from build123d import *

# Parameters (mm, degrees)
SKIZZE1_W                               = 80
SKIZZE1_H                               = 46
SKIZZE1_R                               = 5
SKIZZE1_R_2                             = 1
AUFSATZ_LINEAR_AUSTRAGEN1_DEPTH         = 3
AUFSATZ_LINEAR_AUSTRAGEN1_DEPTH_BACK    = 3
F_3_0_3_DURCHMESSER_BOHRUNG1_AT_2_COUNT = 2
F_3_0_3_DURCHMESSER_BOHRUNG1_AT_2_PITCH = 40
SKIZZE4_W                               = 32
SKIZZE4_H                               = 46
SCHNITT_LINEAR_AUSTRAGEN1_DEPTH         = 4
SCHNITT_LINEAR_AUSTRAGEN3_DEPTH         = 4.5
SKIZZE9_W                               = 35.5
SKIZZE9_H                               = 44
SCHNITT_LINEAR_AUSTRAGEN5_DEPTH         = 2
AUFSATZ_LINEAR_AUSTRAGEN2_DEPTH         = 34
FASE1_SIZE                              = 0.7


with BuildPart() as part:
    # Skizze1 → Aufsatz-Linear austragen1 (new body, two sides)
    with BuildSketch(Plane.XY) as aufsatz_linear_austragen1_sk:
        Rectangle(SKIZZE1_W, SKIZZE1_H)
        with Locations((0, -12)):
            Circle(SKIZZE1_R, mode=Mode.SUBTRACT)
        with Locations((0, -2)):
            Circle(SKIZZE1_R_2, mode=Mode.SUBTRACT)
    extrude(amount=AUFSATZ_LINEAR_AUSTRAGEN1_DEPTH)
    extrude(aufsatz_linear_austragen1_sk.sketch, amount=-AUFSATZ_LINEAR_AUSTRAGEN1_DEPTH_BACK)

    # Skizze2 → Ø3.0 (3) Durchmesser Bohrung1 (revolve, cut)
    with BuildSketch(Plane(origin=(40, -20, 0), x_dir=(0, 0, -1), z_dir=(0, 1, 0))):
        Polygon((0, 0), (0, 12.901290929), (1.5, 12), (1.5, 0), align=None)
    f_3_0_3_durchmesser_bohrung1 = revolve(axis=Axis((46.35, -20, 0), (-1, 0, 0)), mode=Mode.SUBTRACT)

    # Ø3.0 (3) Durchmesser Bohrung1 at 2: Ø3.0 (3) Durchmesser Bohrung1 ×2
    with Locations(*[(0, i * F_3_0_3_DURCHMESSER_BOHRUNG1_AT_2_PITCH, 0) for i in range(1, F_3_0_3_DURCHMESSER_BOHRUNG1_AT_2_COUNT)]):
        add(f_3_0_3_durchmesser_bohrung1, mode=Mode.SUBTRACT)

    # Spiegeln1: Ø3.0 (3) Durchmesser Bohrung1 across plane
    add(f_3_0_3_durchmesser_bohrung1.mirror(Plane(origin=(0, 0, 0), x_dir=(0, 0, 1), z_dir=(1, 0, 0))), mode=Mode.SUBTRACT)

    # Spiegeln1 copy 1 sketch → Spiegeln1 copy 1 (revolve, cut)
    with BuildSketch(Plane(origin=(-40, 20, 0), x_dir=(0, 0, -1), z_dir=(0, 1, 0))):
        Polygon((0, 0), (0, -12.901290929), (1.5, -12), (1.5, 0), align=None)
    revolve(axis=Axis((-46.35, 20, 0), (-1, 0, 0)), mode=Mode.SUBTRACT)

    # Skizze4 → Schnitt-Linear austragen1 (cut)
    with BuildSketch(Plane.XY.offset(-3)):
        Rectangle(SKIZZE4_W, SKIZZE4_H)
    extrude(amount=SCHNITT_LINEAR_AUSTRAGEN1_DEPTH, mode=Mode.SUBTRACT)

    # Skizze6 → Schnitt-Linear austragen3 (cut)
    with BuildSketch(Plane(origin=(0, 0, -3), x_dir=(-1, 0, 0), z_dir=(0, 0, -1))):
        with BuildLine():
            Line((37, 15), (37, -15))
            ThreePointArc((37, -15), (36.414213562, -16.414213562), (35, -17))
            Line((35, -17), (22, -17))
            ThreePointArc((22, -17), (20.585786438, -16.414213562), (20, -15))
            Line((20, -15), (20, 15))
            ThreePointArc((20, 15), (20.585786438, 16.414213562), (22, 17))
            Line((22, 17), (35, 17))
            ThreePointArc((35, 17), (36.414213562, 16.414213562), (37, 15))
        make_face()
        with BuildLine():
            Line((-35, 17), (-22, 17))
            ThreePointArc((-22, 17), (-20.585786438, 16.414213562), (-20, 15))
            Line((-20, 15), (-20, -15))
            ThreePointArc((-20, -15), (-20.585786438, -16.414213562), (-22, -17))
            Line((-22, -17), (-35, -17))
            ThreePointArc((-35, -17), (-36.414213562, -16.414213562), (-37, -15))
            Line((-37, -15), (-37, 15))
            ThreePointArc((-37, 15), (-36.414213562, 16.414213562), (-35, 17))
        make_face()
    extrude(amount=-SCHNITT_LINEAR_AUSTRAGEN3_DEPTH, mode=Mode.SUBTRACT)

    # Skizze9 → Schnitt-Linear austragen5 (cut)
    with BuildSketch(Plane(origin=(0, 0, -3), x_dir=(-1, 0, 0), z_dir=(0, 0, -1))):
        with Locations((0, -1)):
            Rectangle(SKIZZE9_W, SKIZZE9_H)
    extrude(amount=-SCHNITT_LINEAR_AUSTRAGEN5_DEPTH, mode=Mode.SUBTRACT)

    # Skizze10 → Aufsatz-Linear austragen2 (add)
    with BuildSketch(Plane(origin=(0, 23, 0), x_dir=(1, 0, 0), z_dir=(0, 1, 0))):
        Polygon((-16, 3), (-16, 4.5), (-18, 4.5), (-20, 3), align=None)
        Polygon((20, 3), (16, 3), (16, 4.5), (18, 4.5), align=None)
    extrude(amount=-AUFSATZ_LINEAR_AUSTRAGEN2_DEPTH)

    # Fase1
    fase1_edges = [part.edges().sort_by_distance(p)[0] for p in [
        (40, 20, 1.5),
        (40, -20, 1.5),
        (-40, 20, 1.5),
        (-40, -20, 1.5),
    ]]
    chamfer(fase1_edges, length=FASE1_SIZE)


solid = part.part
Part model, mm, in its own coordinate system. A direction names the side the tool comes from. Coordinates: 2 decimals unless noted, no trailing zeros. Loops run counter-clockwise (first coordinate to the right, second up) from the corner with the lowest first, then second, coordinate; pieces in that order, holes last. Notation, with made-up numbers: (-29, 21.5) - (-17, 21.5) arc R34 ccw to (-17, 53.5) - close; hole circle Ø2 at (-8.75, 13.5). An arc over 180 degrees is marked (long way). Write each question's results on one line, items separated by ' | '. Start each with the question number.
Q1. Slice it at C-C on y = 0.5. Give the cut face in (x, z).
Q2. Which spindle directions (+Z, -Z, +X, -X, +Y, -Y) get a long thin tool onto all of the face, cutting with end or side? Do faces 1 (the cylindrical face through (36.4, -16.43, -0.78)), 2 (the flat face through (0, 0, 1)), 3 (the flat face through (-17, 21, -2)), 4 (the cylindrical face through (-33.729, 18.513, 0.195)). Say none if no direction does.
Q3. Two-plate mould, pull along Y, no slides. Class faces 5 (the flat face through (-1, 23, 2)), 6 (the cylindrical face through (36.43, 16.4, -0.78)), 7 (the flat face through (-37.2, 0.1, -3)), 8 (the flat face through (-18, -11, -4)): +Y half, -Y half, draft (parallel to the pull), parting line (faces both ways), or undercut.
Q4. Drop flat-ended pins along their axis: pin 1 Ø18.5 at (x, y) = (-25.5, 5.5) entering from -Z; pin 2 Ø2.5 at (y, z) = (20, 0) entering from +X; pin 3 Ø8 at (x, y) = (-26.5, -9) entering from -Z; pin 4 Ø18.5 at (x, y) = (32.5, -2) entering from -Z. Give the stop position or say it passes through.
Q5. Slice it at B-B on y = -12. Give the cut face in (x, z), and give its area (3 significant figures).
Q6. Slice it at A-A on x = 0. Give the cut face in (y, z).
Q7. Probe line 1 along Y through (x, z) = (34, 0); line 2 along X through (y, z) = (5, -2); line 3 along X through (y, z) = (7.5, 0.5). List the from-to ranges inside material, lowest first.
Q8. Slice it at D-D on x = -23.5. Give the cut face in (y, z), and give its area (3 significant figures).
Answer:
1) outline: (-40, -3) - (-37, -3) - (-37, 1.5) - (-20, 1.5) - (-20, -3) - (-18, -4.5) - (-16, -4.5) - (-16, -3) - (-17.75, -3) - (-17.75, -1) - (-16, -1) - (-16, 1) - (16, 1) - (16, -1) - (17.75, -1) - (17.75, -3) - (16, -3) - (16, -4.5) - (18, -4.5) - (20, -3) - (20, 1.5) - (37, 1.5) - (37, -3) - (40, -3) - (40, 3) - (-40, 3) - close
2) face 1: -Z | face 2: -Z, +Y, -Y | face 3: -Y | face 4: -X
3) face 5: +Y half | face 6: undercut | face 7: draft | face 8: -Y half
4) pin 1: stops at z = -4.5 | pin 2: stops at x = 27.85 | pin 3: stops at z = 1.5 | pin 4: stops at z = -3
5) outline: (-40, -3) - (-37, -3) - (-37, 1.5) - (-20, 1.5) - (-20, -3) - (-17.75, -3) - (-17.75, -1) - (-16, -1) - (-16, 1) - (-5, 1) - (-5, 3) - (-40, 3) - close; (5, 1) - (16, 1) - (16, -1) - (17.75, -1) - (17.75, -3) - (20, -3) - (20, 1.5) - (37, 1.5) - (37, -3) - (40, -3) - (40, 3) - (5, 3) - close | area: 172 mm2
6) outline: (-23, 1) - (-17, 1) - (-17, 3) - (-23, 3) - close; (-7, 1) - (-3, 1) - (-3, 3) - (-7, 3) - close; (-1, 1) - (23, 1) - (23, 3) - (-1, 3) - close
7) line 1: y = -23 to -21.5, -18.5 to -17, 17 to 18.5, 21.5 to 23 | line 2: x = -40 to -37, -20 to -17.75, 17.75 to 20, 37 to 40 | line 3: x = -40 to -37, -20 to -16, 16 to 20, 37 to 40
8) outline: (-23, -3) - (-17, -3) - (-17, 1.5) - (17, 1.5) - (17, -3) - (23, -3) - (23, 3) - (-23, 3) - close | area: 123 mm2
